Can you work these out from the model? Positions are in its coordinate system, mm. A direction names the side the tool comes from. Round coordinates to 2 decimals unless told otherwise and drop trailing zeros. Loops run counter-clockwise (first coordinate to the right, second up) from the corner with the lowest first, then second, coordinate; pieces in that order, holes last.
(1) Will these pins go through, and if not, where does the flat tip stop? pin 1 Ø3 at (x, z) = (68.5, -8) entering from -Y; pin 2 Ø1.5 at (x, y) = (37.5, 14.5) entering from -Z; pin 3 Ø10 at (x, z) = (33.5, -26.5) entering from +Y.
(2) I want a section at B-B on z = -42. Write out the boundary of the cut face in (x, y), plus the area to 3 significant figures.
(3) Thinking about a two-plate mould opening in X: for faces 1 (the face through (2, 25, -3)), 2 (the face through (38, 29, -5)), 3 (the face through (72, 25, -33)), which applies, released by +X, released by -X, zero draft, split by the parting line, or undercut?
(4) If I drill on line 1 along X through (y, z) = (6, -8); line 2 along X through (y, z) = (19.5, -30); line 3 along Y through (x, z) = (49, -2.3), over which ranges is the centre line in solid material (lowest first)?
(5) I want a section at D-D on x = 16. Write out the boundary of the cut face in (y, z).
(6) I want a section at C-C on y = 6.5. Write out the boundary of the cut face in (x, z), plus the area to 3 significant figures.
(7) I want a section at A-A on y = 27.5. Write out the boundary of the cut face in (x, z).
(8) Which directions (+Z, -Z, +X, -X, +Y, -Y) give clear straight access to the entire face, cutting with the end or side of a thin tool? Please do faces 4 (the face through (7, 10, -42)), 5 (the face through (61, 24, -17)), 6 (the face through (72, 25, -2)).
from build123d import *
from OCP.BRepFilletAPI import BRepFilletAPI_MakeChamfer

# Parameters (mm, degrees)
SKETCH1_W           = 75
SKETCH1_H           = 17
BOSS_EXTRUDE1_DEPTH = 50
SKETCH2_W           = 12
SKETCH2_H           = 25
BOSS_EXTRUDE2_DEPTH = 38
SKETCH3_W           = 75
SKETCH3_H           = 55
BOSS_EXTRUDE3_DEPTH = 8
SKETCH4_R           = 2.5
CUT_EXTRUDE1_DEPTH  = 10
SKETCH5_W           = 40
SKETCH5_H           = 42
CUT_EXTRUDE2_DEPTH  = 12
CUT_EXTRUDE3_DEPTH  = 104.07764064
CHAMFER1_SIZE       = 5
CHAMFER3_SIZE       = 5
CHAMFER3_SIZE_2     = 10
CHAMFER4_SIZE       = 5
CHAMFER4_SIZE2      = 10


with BuildPart() as part:
    # Sketch1 → Boss-Extrude1 (new body)
    with BuildSketch(Plane(origin=(0, 0, 0), x_dir=(1, 0, 0), z_dir=(0, 1, 0))):
        with Locations((37.5, 8.5)):
            Rectangle(SKETCH1_W, SKETCH1_H)
    extrude(amount=BOSS_EXTRUDE1_DEPTH)

    # Sketch2 → Boss-Extrude2 (add)
    with BuildSketch(Plane(origin=(0, 0, -17), x_dir=(-1, 0, 0), z_dir=(0, 0, -1))):
        with Locations((-69, 12.5)):
            Rectangle(SKETCH2_W, SKETCH2_H)
        with Locations((-6, 12.5)):
            Rectangle(SKETCH2_W, SKETCH2_H)
    extrude(amount=BOSS_EXTRUDE2_DEPTH)

    # Sketch3 → Boss-Extrude3 (add)
    with BuildSketch(Plane.XZ):
        with Locations((37.5, -27.5)):
            Rectangle(SKETCH3_W, SKETCH3_H)
    extrude(amount=-BOSS_EXTRUDE3_DEPTH)

    # Sketch4 → Cut-Extrude1 (cut)
    with BuildSketch(Plane(origin=(0, 0, 0), x_dir=(-1, 0, 0), z_dir=(0, -1, 0))):
        with Locations(Location((-6.5, 8, 0), (0, 0, 90))):
            Circle(SKETCH4_R)
        with Locations(Location((-68.5, 8, 0), (0, 0, 90))):
            Circle(SKETCH4_R)
        with Locations(Location((-6.5, 42, 0), (0, 0, 90))):
            Circle(SKETCH4_R)
        with Locations(Location((-68.5, 42, 0), (0, 0, 90))):
            Circle(SKETCH4_R)
    extrude(amount=-CUT_EXTRUDE1_DEPTH, mode=Mode.SUBTRACT)

    # Sketch5 → Cut-Extrude2 (cut)
    with BuildSketch(Plane(origin=(0, 0, -17), x_dir=(-1, 0, 0), z_dir=(0, 0, -1))):
        with Locations((-37.5, 29)):
            Rectangle(SKETCH5_W, SKETCH5_H)
    extrude(amount=-CUT_EXTRUDE2_DEPTH, mode=Mode.SUBTRACT)

    # Sketch6 → Cut-Extrude3 (cut, through all)
    with BuildSketch(Plane(origin=(0, 0, -5), x_dir=(-1, 0, 0), z_dir=(0, 0, -1))):
        with BuildLine():
            Line((-49, 39.5), (-49, 42))
            Line((-49, 42), (-46.5, 42))
            ThreePointArc((-46.5, 42), (-50.767766953, 43.767766953), (-49, 39.5))
        make_face()
        with BuildLine():
            Line((-46.5, 42), (-49, 42))
            Line((-49, 42), (-49, 39.5))
            ThreePointArc((-49, 39.5), (-47.232233047, 40.232233047), (-46.5, 42))
        make_face()
        with BuildLine():
            ThreePointArc((-23.5, 19), (-24.232233047, 20.767766953), (-26, 21.5))
            Line((-26, 21.5), (-26, 19))
            Line((-26, 19), (-28.5, 19))
            ThreePointArc((-28.5, 19), (-26, 16.5), (-23.5, 19))
        make_face()
        with BuildLine():
            Line((-26, 19), (-26, 21.5))
            ThreePointArc((-26, 21.5), (-27.767766953, 20.767766953), (-28.5, 19))
            Line((-28.5, 19), (-26, 19))
        make_face()
    extrude(amount=-CUT_EXTRUDE3_DEPTH, mode=Mode.SUBTRACT)

    # Chamfer1
    chamfer1_edges = [part.edges().sort_by_distance(p)[0] for p in [
        (63, 25, -36),
        (12, 25, -36),
        (75, 25, 0),
        (0, 25, 0),
    ]]
    chamfer(chamfer1_edges, length=CHAMFER1_SIZE)

    # Chamfer3
    chamfer3_edges_1 = [part.edges().sort_by_distance(p)[0] for p in [
        (0, 37.5, -17),
    ]]
    chamfer3_side_1 = [part.faces().sort_by_distance(p)[0] for p in [
        (0, 37.5, -16.9),
    ]]
    chamfer3_edges_2 = [part.edges().sort_by_distance(p)[0] for p in [
        (8.75, 50, -17),
    ]]
    chamfer3_side_2 = [part.faces().sort_by_distance(p)[0] for p in [
        (8.75, 50, -16.9),
    ]]
    chamfer3 = BRepFilletAPI_MakeChamfer(part.part.solid().wrapped)
    for e in chamfer3_edges_1:
        chamfer3.Add(CHAMFER3_SIZE - 0.0001, CHAMFER3_SIZE_2 - 0.0001, e.wrapped, chamfer3_side_1[0].wrapped)
    for e in chamfer3_edges_2:
        chamfer3.Add(CHAMFER3_SIZE - 0.0001, CHAMFER3_SIZE_2 - 0.0001, e.wrapped, chamfer3_side_2[0].wrapped)
    add(Compound.cast(chamfer3.Shape()), mode=Mode.REPLACE)  # a hair under: the kernel refuses the full size

    # Chamfer4: one chamfer whose edges measure the first distance from different faces: ONE call of the kernel's chamfer builder (chamfer() names one face for all edges)
    chamfer4_edges_1 = [part.edges().sort_by_distance(p)[0] for p in [
        (66.25, 50, -17),
    ]]
    chamfer4_side_1 = [part.faces().sort_by_distance(p)[0] for p in [
        (0.769025357, 50, -8.50005),
    ]]
    chamfer4_edges_2 = [part.edges().sort_by_distance(p)[0] for p in [
        (75, 37.5, -17),
    ]]
    chamfer4_side_2 = [part.faces().sort_by_distance(p)[0] for p in [
        (75, 17.338709677, -26.322580645),
    ]]
    chamfer4 = BRepFilletAPI_MakeChamfer(part.part.solid().wrapped)
    for e in chamfer4_edges_1:
        chamfer4.Add(CHAMFER4_SIZE, CHAMFER4_SIZE2, e.wrapped, chamfer4_side_1[0].wrapped)  # the first distance lies on this face
    for e in chamfer4_edges_2:
        chamfer4.Add(CHAMFER4_SIZE, CHAMFER4_SIZE2, e.wrapped, chamfer4_side_2[0].wrapped)  # the first distance lies on this face
    add(Compound.cast(chamfer4.Shape()), mode=Mode.REPLACE)


solid = part.part
Filled sheet:
1. pin 1: stops at y = 10
1. pin 2: stops at z = -5
1. pin 3: stops at y = 8
2. outline: (0, 0) - (4, 0) - (4, 10) - (9, 10) - (9, 0) - (66, 0) - (66, 10) - (71, 10) - (71, 0) - (75, 0) - (75, 25) - (68, 25) - (63, 20) - (63, 8) - (12, 8) - (12, 20) - (7, 25) - (0, 25) - close
2. area: 883 mm2
3. face 1: released by -X
3. face 2: undercut
3. face 3: zero draft
4. line 1: x = 0 to 4, 9 to 66, 71 to 75
4. line 2: x = 0 to 12, 63 to 75
4. line 3: y = 0 to 39.5, 44.5 to 50
5. outline: (0, -55) - (8, -55) - (8, -17) - (40, -17) - (50, -12) - (50, 0) - (0, 0) - close
6. outline: (0, -55) - (75, -55) - (75, -5) - (70, 0) - (5, 0) - (0, -5) - close; hole circle Ø5 at (6.5, -42); hole circle Ø5 at (6.5, -8); hole circle Ø5 at (68.5, -42); hole circle Ø5 at (68.5, -8)
6. area: 4,020 mm2
7. outline: (0, -12) - (10, -17) - (17.5, -17) - (17.5, -5) - (57.5, -5) - (57.5, -17) - (65, -17) - (75, -12) - (75, -5) - (70, 0) - (5, 0) - (0, -5) - close
8. face 4: -Y
8. face 5: -Z, +Y
8. face 6: +Z, +X, +Y, -Y
